Input: part model. Units: mm. Frame: model coordinates. Face numbers are marked on the shaded views. A direction names the side the tool comes from. Coordinates: 2 decimals unless noted, no trailing zeros. Write each loop counter-clockwise with the first axis right and the second up, starting at its lowest first coordinate (ties: lowest second). Pieces come first, ordered by that corner, then holes. Notation, with made-up numbers: (11, 11.5) - (30, 11.5) arc R12 cw to (30, 16.5) - close; hole circle Ø9 at (4, 23). An arc over 180 degrees is marked (long way). Put each result on its own line as item: value. Start each with the question number.
1. Cut plane A-A, the plane x = 15. Return loops of the section in (y, z) (3 decimals).
2. Cut plane D-D, the plane z = 44.5. Return loops of the section in (x, y) (3 decimals).
3. Cut plane B-B, the plane y = 14. Return loops of the section in (x, z) (3 decimals), and give its area (3 significant figures).
4. Access query for the marked faces 1 and 2. Directions: +Z, -Z, +X, -X, +Y, -Y. A direction counts if a zero-diameter tool reaches every point of the face in a straight line with its end or side. Return the directions, or none.
5. Cut plane C-C, the plane z = 3.81. Return loops of the section in (x, y) (3 decimals), and give its area (3 significant figures).
6. Pin query (flat end, axial travel): pin 1 (4 mm diameter, centred on x = 6, y = 33, fed in from +Z); pin 2 (3 mm diameter, centred on x = 22, z = 62.5, fed in from +Y) (3 decimals); pin 3 (12 mm diameter, centred on x = 8, z = 70.5, fed in from +Y); pin 4 (3 mm diameter, centred on y = 12.5, z = 75.5, fed in from +X) (3 decimals). Return the tip coordinate at first contact, or that it passes through.
7. Line query: line 1 (Z direction, x = 17, y = 3) (3 decimals); line 2 (X direction, y = 29, z = 109.5) (3 decimals). Output: solid intervals per line, ascending.
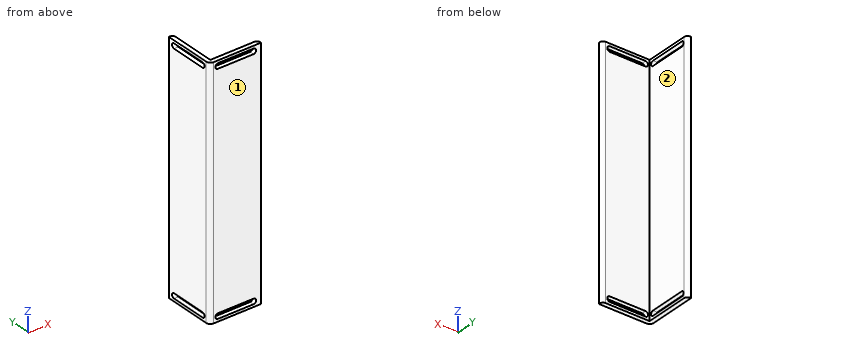
from build123d import *

# Parameters (mm, degrees)
BOSS_EXTRUDE1_DEPTH = 177.8
FILLET1_R           = 3.175
CUT_EXTRUDE2_DEPTH  = 177.8
CUT_EXTRUDE6_DEPTH  = 177.8


with BuildPart() as part:
    # Sketch1 → Boss-Extrude1 (new body)
    with BuildSketch(Plane.XY):
        with BuildLine():
            Line((0, 0), (0, 38.1))
            Line((0, 38.1), (0.635, 38.1))
            ThreePointArc((0.635, 38.1), (2.431051224, 37.356051224), (3.175, 35.56))
            Line((3.175, 35.56), (3.175, 3.175))
            Line((3.175, 3.175), (35.56, 3.175))
            ThreePointArc((35.56, 3.175), (37.356051224, 2.431051224), (38.1, 0.635))
            Line((38.1, 0.635), (38.1, 0))
            Line((38.1, 0), (0, 0))
        make_face()
    extrude(amount=BOSS_EXTRUDE1_DEPTH)

    # Fillet1
    fillet1_edges = [part.edges().sort_by_distance(p)[0] for p in [
        (0, 0, 88.9),
    ]]
    fillet(fillet1_edges, radius=FILLET1_R)

    # Sketch2 → Cut-Extrude2 (cut)
    with BuildSketch(Plane(origin=(3.175, 0, 0), x_dir=(0, 0, -1), z_dir=(1, 0, 0))):
        with BuildLine():
            Line((-172.101028795, 33.266000832), (-172.101028795, 6.35722327))
            ThreePointArc((-172.101028795, 6.35722327), (-173.92929525, 4.528956814), (-175.757561706, 6.35722327))
            Line((-175.757561706, 6.35722327), (-175.757561706, 33.266000832))
            ThreePointArc((-175.757561706, 33.266000832), (-173.92929525, 35.094267287), (-172.101028795, 33.266000832))
        make_face()
        with BuildLine():
            Line((-5.698971205, 33.266000832), (-5.698971205, 6.35722327))
            ThreePointArc((-5.698971205, 6.35722327), (-3.87070475, 4.528956814), (-2.042438294, 6.35722327))
            Line((-2.042438294, 6.35722327), (-2.042438294, 33.266000832))
            ThreePointArc((-2.042438294, 33.266000832), (-3.87070475, 35.094267287), (-5.698971205, 33.266000832))
        make_face()
    extrude(amount=-CUT_EXTRUDE2_DEPTH, mode=Mode.SUBTRACT)

    # Sketch6 → Cut-Extrude6 (cut)
    with BuildSketch(Plane.XZ):
        with BuildLine():
            Line((32.490336277, 175.895), (6.232036019, 175.895))
            ThreePointArc((6.232036019, 175.895), (4.327036019, 173.99), (6.232036019, 172.085))
            Line((6.232036019, 172.085), (32.490336277, 172.085))
            ThreePointArc((32.490336277, 172.085), (34.395336277, 173.99), (32.490336277, 175.895))
        make_face()
        with BuildLine():
            ThreePointArc((6.232036019, 1.905), (4.327036019, 3.81), (6.232036019, 5.715))
            Line((6.232036019, 5.715), (32.490336277, 5.715))
            ThreePointArc((32.490336277, 5.715), (34.395336277, 3.81), (32.490336277, 1.905))
            Line((32.490336277, 1.905), (6.232036019, 1.905))
        make_face()
    extrude(amount=-CUT_EXTRUDE6_DEPTH, mode=Mode.SUBTRACT)


solid = part.part
Report:
1. outline: (0, 0) - (3.175, 0) - (3.175, 1.905) - (0, 1.905) - close; (0, 5.715) - (3.175, 5.715) - (3.175, 172.085) - (0, 172.085) - close; (0, 175.895) - (3.175, 175.895) - (3.175, 177.8) - (0, 177.8) - close
2. outline: (0, 3.175) arc R3.175 ccw to (3.175, 0) - (38.1, 0) - (38.1, 0.635) arc R2.54 ccw to (35.56, 3.175) - (3.175, 3.175) - (3.175, 35.56) arc R2.54 ccw to (0.635, 38.1) - (0, 38.1) - close
3. outline: (0, 0) - (3.175, 0) - (3.175, 2.042) - (0, 2.042) - close; (0, 5.699) - (3.175, 5.699) - (3.175, 172.101) - (0, 172.101) - close; (0, 175.758) - (3.175, 175.758) - (3.175, 177.8) - (0, 177.8) - close
3. area: 541 mm^2
4. face 1: +Z, -Z, +X, -X, -Y
4. face 2: +Z, -Z, +X, +Y
5. outline: (0, 3.175) arc R3.175 ccw to (3.175, 0) - (4.327, 0) - (4.327, 3.175) - (3.175, 3.175) - (3.175, 4.53) - (0, 4.53) - close; (0, 35.093) - (3.175, 35.093) - (3.175, 35.56) arc R2.54 ccw to (0.635, 38.1) - (0, 38.1) - close; (34.395, 0) - (38.1, 0) - (38.1, 0.635) arc R2.54 ccw to (35.56, 3.175) - (34.395, 3.175) - close
5. area: 34.4 mm^2
6. pin 1: passes through
6. pin 2: stops at y = 3.175
6. pin 3: stops at y = 37.7
6. pin 4: stops at x = 3.175
7. line 1: z = 0 to 1.905, 5.715 to 172.085, 175.895 to 177.8
7. line 2: x = 0 to 3.175
